from build123d import *

# Parameters (mm, degrees)
F1_DEPTH = 15
F3_DEPTH = 25


# Not quite as in the source:
# - a pattern or mirror of a feature is missing from the dataset's text; its kind, count and spacing are read off the source's solid


with BuildPart() as f1:
    # F0 (on Front) → F1 (new body, symmetric)
    with BuildSketch(Plane.XZ):
        with BuildLine():
            ThreePointArc((11.9895788083, -27.5), (25.0966866762, -16.4364326384), (30, 0))
            ThreePointArc((30, 0), (25.0966866762, 16.4364326384), (11.9895788083, 27.5))
            Line((11.9895788083, 27.5), (-11.9895788083, 27.5))
            ThreePointArc((-11.9895788083, 27.5), (-30, 0), (-11.9895788083, -27.5))
            Line((-11.9895788083, -27.5), (11.9895788083, -27.5))
        make_face()
    extrude(amount=F1_DEPTH, both=True)

    # F2 (on face) → F3 (join)
    with BuildSketch(Plane.XZ.offset(15)):
        with BuildLine():
            ThreePointArc((7.5, -21.2132034356), (18.3711730709, -12.9903810568), (22.5, 0))
            ThreePointArc((22.5, 0), (18.3711730709, 12.9903810568), (7.5, 21.2132034356))
            Line((7.5, 21.2132034356), (7.5, 12.5))
            Line((7.5, 12.5), (-7.5, 12.5))
            Line((-7.5, 12.5), (-7.5, 21.2132034356))
            ThreePointArc((-7.5, 21.2132034356), (-22.5, 0), (-7.5, -21.2132034356))
            Line((-7.5, -21.2132034356), (-7.5, -12.5))
            Line((-7.5, -12.5), (7.5, -12.5))
            Line((7.5, -12.5), (7.5, -21.2132034356))
        make_face()
    f3 = extrude(amount=F3_DEPTH)

    # F3_copies: F3 across plane
    add(f3.mirror(Plane.ZX))


solid = f1.part
The listing builds one solid part. Answer for the finished solid, in the listing's coordinates (mm). A direction names the side the tool comes from. Give positions to 0.01 mm unless a question says otherwise; leave off trailing zeros. Write each loop counter-clockwise with the first axis right and the second up, starting at its lowest first coordinate (ties: lowest second). Pieces come first, ordered by that corner, then holes. Notation, with made-up numbers: (-23, 16) - (-16, 16) arc R14 ccw to (-16, 38) - close; hole circle Ø6 at (58.25, 68.5). An arc over 180 degrees is marked (long way). Use a Markdown table: item, result.
1. For a pull along X with two mould halves and no side action, classify faces 5 (the flat face through (0, -27, -12.5)), 6 (the flat face through (0, -40, 0)), 7 (the cylindrical face through (-22.497, -27.325, 0.388)) as released by +X, released by -X, zero draft, split by the parting line, or undercut.
Values follow:
| item | result |
|---|---|
| face 5 | undercut |
| face 6 | zero draft |
| face 7 | released by -X |
2. A tool of negligible diameter and unlimited length cuts with its end or side. For faces 1 (the flat face through (7.5, 27, 17)), 2 (the flat face through (7.5, -27, 17)), 3 (the flat face through (-7.5, -27, -17)), 4 (the flat face through (-7.5, 27, -17)), from which of +Z, -Z, +X, -X, +Y, -Y can it reach the whole face along a straight path? Write none if from no direction.
Values follow:
| item | result |
|---|---|
| face 1 | +Z, +Y |
| face 2 | +Z, -Y |
| face 3 | -Z, -Y |
| face 4 | -Z, +Y |
3. Section C-C on z = -6 is taken. Write down the section's boundary in (x, y), plus the area to 3 significant figures.
Values follow:
| item | result |
|---|---|
| outline | (-29.39, -15) - (-21.69, -15) - (-21.69, -40) - (21.69, -40) - (21.69, -15) - (29.39, -15) - (29.39, 15) - (21.69, 15) - (21.69, 40) - (-21.69, 40) - (-21.69, 15) - (-29.39, 15) - close |
| area | 3,930 mm² |
4. Section A-A on y = -23 is taken. Write down the section's boundary in (x, z), plus the area to 3 significant figures.
Values follow:
| item | result |
|---|---|
| outline | (-7.5, -21.21) - (-7.5, -12.5) - (7.5, -12.5) - (7.5, -21.21) arc R22.5 ccw to (7.5, 21.21) - (7.5, 12.5) - (-7.5, 12.5) - (-7.5, 21.21) arc R22.5 ccw to start |
| area | 1,300 mm² |
5. Each of these flat-tipped pins is pushed along its axis until it touches: P1, Ø3, axis at y = -19, z = 0.5, coming from the +X side; P2, Ø12, axis at x = -0.5, y = -28.5, coming from the -Z side; P3, Ø4.5, axis at y = 23.5, z = -18.5, coming from the +X side. Where does it stop, or does it pass through?
Values follow:
| item | result |
|---|---|
| P1 | stops at x = 22.5 |
| P2 | stops at z = -12.5 |
| P3 | stops at x = 15.56 |
6. Find the intervals of material crossed by probe 1 along Y at (x, z) = (-5, 25); probe 2 along Z at (x, y) = (5, -15.5); probe 3 along X at (y, z) = (20.5, 17), in increasing order. Write a range as from..to.
Values follow:
| item | result |
|---|---|
| probe 1 | y = -15..15 |
| probe 2 | z = -12.5..12.5 |
| probe 3 | x = -14.74..-7.5, 7.5..14.74 |
7. Section D-D on z = -13.5 is taken. Write down the section's boundary in (x, y), plus the area to 3 significant figures.
Values follow:
| item | result |
|---|---|
| outline | (-26.79, -15) - (-18, -15) - (-18, -40) - (-7.5, -40) - (-7.5, -15) - (7.5, -15) - (7.5, -40) - (18, -40) - (18, -15) - (26.79, -15) - (26.79, 15) - (18, 15) - (18, 40) - (7.5, 40) - (7.5, 15) - (-7.5, 15) - (-7.5, 40) - (-18, 40) - (-18, 15) - (-26.79, 15) - close |
| area | 2,660 mm² |
8. Section B-B on x = -15 is taken. Write down the section's boundary in (y, z), plus the area to 3 significant figures.
Values follow:
| item | result |
|---|---|
| outline | (-40, -16.77) - (-15, -16.77) - (-15, -25.98) - (15, -25.98) - (15, -16.77) - (40, -16.77) - (40, 16.77) - (15, 16.77) - (15, 25.98) - (-15, 25.98) - (-15, 16.77) - (-40, 16.77) - close |
| area | 3,240 mm² |
